Autodesk Inventor part; units mm, degrees
ref_plane "YZ Plane" through (0, 0, 0) normal (1, 0, 0) x (0, 1, 0)
ref_plane "XZ Plane" through (0, 0, 0) normal (0, 1, 0) x (-1, 0, 0)
ref_plane "XY Plane" through (0, 0, 0) normal (0, 0, 1) x (1, 0, 0)
sketch "Sketch1" plane through (0, 0, 0) normal (0, 1, 0) x (-1, 0, 0)
  line L0 (0, 0) -> (34, 0)
  line L1 (34, 0) -> (34, -40)
  line L2 (34, -40) -> (0, -40)
  line L3 (0, -40) -> (0, 0)
  line L4 (17, -40) -> (17, 0)
  line L5 (34, -20) -> (0, -20)
  dimension "d0" = 34
  dimension "d1" = 40
extrude "Extrusion1" add sketch "Sketch1" along normal blind 3
sketch "Sketch2" plane through (0, 3, 0) normal (0, 1, 0) x (1, 0, 0)
  line L0 (-34, 40) -> (-34, 0)
  line L1 (0, 0) -> (0, 40)
  line L2 (0, 40) -> (-34, 40)
  line L3 (-34, 0) -> (0, 0)
  circle A0 centre (-17, 20) radius 9
  line L4 (-34, 0) -> (0, 0)
  line L5 (0, 0) -> (0, 40)
  line L6 (0, 40) -> (-34, 40)
  line L7 (-34, 40) -> (-34, 0)
  dimension "d4" = 18
extrude "Extrusion2" add sketch "Sketch2" along normal blind 2
sketch "Sketch4" plane through (-17, 3, -20) normal (0, 1, 0) x (1, 0, 0)
  line L0 (0, 0) -> (0, 6)
  circle A0 centre (0, 6) radius 2.175
  circle A1 centre (0, -6) radius 2.175
  circle A2 centre (6, 0) radius 2.175
  circle A3 centre (-6, 0) radius 2.175
  point P0 (17, -20)
  dimension "d7" = 6
  dimension "d8" = 4.35
  dimension "d9" = 4.35
  dimension "d10" = 12
  dimension "d11" = 4.35
  dimension "d12" = 6
  dimension "d13" = 4.35
  dimension "d14" = 12
hole "Hole1" at (-23, 3, -20) at (-17, 3, -26) at (-11, 3, -20) at (-17, 3, -14) direction (0, -1, 0) diameter 4.35 end through all
sketch "Sketch5" plane through (0, 5, 0) normal (0, 1, 0) x (1, 0, 0)
  line L0 (0, 0) -> (-7, 0)
  line L1 (-7, 0) -> (-7, 7)
  line L2 (-7, 7) -> (0, 7)
  line L3 (0, 7) -> (0, 0)
  line L4 (0, 40) -> (-7, 40)
  line L5 (-7, 40) -> (-7, 33)
  line L6 (-7, 33) -> (0, 33)
  line L7 (0, 33) -> (0, 40)
  line L8 (0, 40) -> (-34, 40)
  line L9 (-34, 40) -> (-27, 40)
  line L10 (-27, 40) -> (-27, 33)
  line L11 (-27, 33) -> (-34, 33)
  line L12 (-34, 33) -> (-34, 40)
  line L13 (-34, 40) -> (-34, 0)
  line L14 (-34, 0) -> (-27, 0)
  line L15 (-27, 0) -> (-27, 7)
  line L16 (-27, 7) -> (-34, 7)
  line L17 (-34, 7) -> (-34, 0)
  dimension "d22" = 7
  dimension "d23" = 7
  dimension "d24" = 7
  dimension "d25" = 7
extrude "Extrusion3" add sketch "Sketch5" along normal blind 55
sketch "Sketch6" plane through (-34, 0, -40) normal (-1, 0, 0) x (0, 0, 1)
  line L0 (7, 60) -> (0, 60)
  line L1 (0, 60) -> (0, 40)
  line L2 (0, 0) -> (0, 60)
  line L3 (0, 40) -> (40, 60)
  line L4 (40, 60) -> (40, 40)
  line L5 (40, 5) -> (40, 60)
  line L6 (40, 60) -> (0, 60)
  point P0 (40, 0)
  dimension "d28" = 20
extrude "Extrusion4" cut sketch "Sketch6" against normal through all
sketch "Sketch7" plane through (-34, 43.5, -33) normal (0, 0.8944, -0.4472) x (1, 0, 0)
  line L0 (34, -10.0623) -> (34, -36.8951)
  line L1 (0, 25.7148) -> (0, -10.0623)
  line L2 (34, -36.8951) -> (0, -36.8951)
  line L3 (0, -36.8951) -> (0, 7.8262)
  line L4 (0, 7.8262) -> (34, 7.8262)
  line L5 (34, 7.8262) -> (34, -36.8951)
extrude "Extrusion5" add sketch "Sketch7" along normal blind 3
properties part number "cameraMount"
Input: part model. Units: mm. Frame: model coordinates. A direction names the side the tool comes from. Give positions to 0.01 mm unless a question says otherwise; leave off trailing zeros. Order: outer loops, then holes, each group sorted by start corner. A loop starts at its lowest first (then second) coordinate and runs counter-clockwise, first axis right, second up.
1. Cut plane A-A (x = -17). Return loops of the section in (y, z) (3 decimals).
Computed:
outline: (0, -40) - (5, -40) - (5, -29) - (3, -29) - (3, -28.175) - (0, -28.175) - close; (0, -23.825) - (3, -23.825) - (3, -16.175) - (0, -16.175) - close; (0, -11.825) - (3, -11.825) - (3, -11) - (5, -11) - (5, 0) - (0, 0) - close; (40, -40) - (42.683, -41.342) - (62.683, -1.342) - (60, 0) - close
2. Cut plane D-D (x = -12). Return loops of the section in (y, z).
Computed:
outline: (0, -40) - (5, -40) - (5, -27.48) - (3, -27.48) - (3, -21.93) - (0, -21.93) - close; (0, -18.07) - (3, -18.07) - (3, -12.52) - (5, -12.52) - (5, 0) - (0, 0) - close; (40, -40) - (42.68, -41.34) - (62.68, -1.34) - (60, 0) - close
3. Line query: probe 1 along X at (y, z) = (1, -20) (3 decimals); probe 2 along X at (y, z) = (50.5, -2.5); probe 3 along Z at (x, y) = (-17, 4). Output: solid intervals per line, ascending.
Computed:
probe 1: x = -34 to -25.175, -20.825 to -13.175, -8.825 to 0
probe 2: x = -34 to -27, -7 to 0
probe 3: z = -40 to -29, -11 to 0
4. Set-up query: faces 1 (the face through (-27, 32, -3)), 2 (the face through (-17, 50, -20)), 3 (the face through (-17.096, 1.479, -16.173)). Return all of +Z, -Z, +X, -X, +Y, -Y with unobstructed straight access to the full face (end or side cutting, diameter ignored); none if empty.
Computed:
face 1: +Z
face 2: none
face 3: -Y
5. Cut plane C-C (z = -32). Return loops of the section in (x, y), and give its area (3 significant figures).
Computed:
outline: (-34, 0) - (0, 0) - (0, 5) - (-34, 5) - close; (-34, 44) - (0, 44) - (0, 47.35) - (-34, 47.35) - close
area: 284 mm2
6. Draft query along Y for faces 4 (the face through (-24.47, 1.479, -21.603)), 5 (the face through (-17.238, 52.543, -21.622)), 6 (the face through (-8.416, 3.986, -17.297)). Return one class per face: released by +Y, released by -Y, zero draft, split by the parting line, or undercut.
Computed:
face 4: zero draft
face 5: released by +Y
face 6: undercut
7. Cut plane B-B (y = 15). Return loops of the section in (x, z).
Computed:
outline: (-34, -40) - (-27, -40) - (-27, -33) - (-34, -33) - close; (-34, -7) - (-27, -7) - (-27, 0) - (-34, 0) - close; (-7, -40) - (0, -40) - (0, -33) - (-7, -33) - close; (-7, -7) - (0, -7) - (0, 0) - (-7, 0) - close
8. Pin query (flat end, axial travel): pin 1 Ø2.5 at (x, z) = (-17, -14) entering from +Y; pin 2 Ø12 at (y, z) = (50.5, -10) entering from -X; pin 3 Ø12 at (x, z) = (-19, -31) entering from +Y; pin 4 Ø3.5 at (x, z) = (-17, -26) entering from -Y (3 decimals). Return the tip coordinate at first contact, or that it passes through.
Computed:
pin 1: stops at y = 56.98
pin 2: stops at x = -34
pin 3: stops at y = 50.85
pin 4: stops at y = 46.125
